Geometry check sheet. Reference: the model listing, model coordinates, mm. A direction names the side the tool comes from. Round coordinates to 2 decimals unless told otherwise and drop trailing zeros. Order: outer loops, then holes, each group sorted by start corner. A loop starts at its lowest first (then second) coordinate and runs counter-clockwise, first axis right, second up.
(1) Set-up check for faces 1 (the face through (13, -381, -39)), 2 (the face through (13, -193, 0)): record each of +Z, -Z, +X, -X, +Y, -Y from which the full face is reachable in a straight line by a thin tool's end or side.
(2) Release check for a two-part mould opening along Z. For faces 3 (the face through (12.522, -13.668, -42.964)), 4 (the face through (25.4, -168, -37)), 5 (the face through (13, -193, -76.2)) record: +Z half, -Z half, draft (parallel to the pull), parting line (faces both ways), or undercut.
(3) Sectioned sample at A-A (y = -25.4). Record the boundary of the cut face in (x, z), plus the area to 3 significant figures.
(4) Sectioned sample at D-D (z = -88). Record the boundary of the cut face in (x, y), plus the area to 3 significant figures.
(5) Sectioned sample at C-C (x = 14.5). Record the boundary of the cut face in (y, z), plus the area to 3 significant figures.
(6) Go/stop test with flat-tipped pins: pin 1 (12 mm diameter, centred on x = 6.5, y = -10.5, fed in from +Z); pin 2 (10 mm diameter, centred on x = 14, y = -322.5, fed in from -Z). Record where each tip stops, or that it passes through.
(7) Material ranges on line 1 along Z through (x, y) = (19.75, -25.4); line 2 along Z through (x, y) = (3, -243.5); line 3 along Z through (x, y) = (9.75, -14), recorded low to high.
(8) Sectioned sample at B-B (z = -38.1). Record the boundary of the cut face in (x, y), plus the area to 3 significant figures.
from build123d import *

# Parameters (mm, degrees)
F0_W     = 381
F0_H     = 76.2
F0_R     = 12.7
F1_DEPTH = 25.4


with BuildPart() as f1:
    # F0 (on Right) → F1 (new body)
    with BuildSketch(Plane.YZ):
        with Locations((-190.5, -38.1)):
            Rectangle(F0_W, F0_H)
        with Locations((-25.4, -38.1)):
            Circle(F0_R, mode=Mode.SUBTRACT)
        Polygon((50.8, 50.8), (0, 0), (0, -76.2), (50.8, -127), align=None)
    extrude(amount=F1_DEPTH)


solid = f1.part
Answer below:
1. face 1: +Z, -Z, +X, -X, -Y
1. face 2: +Z, +X, -X, -Y
2. face 3: undercut
2. face 4: draft
2. face 5: -Z half
3. outline: (0, -76.2) - (25.4, -76.2) - (25.4, -50.8) - (0, -50.8) - close; (0, -25.4) - (25.4, -25.4) - (25.4, 0) - (0, 0) - close
3. area: 1,290 mm2
4. outline: (0, 11.8) - (25.4, 11.8) - (25.4, 50.8) - (0, 50.8) - close
4. area: 991 mm2
5. outline: (-381, -76.2) - (0, -76.2) - (50.8, -127) - (50.8, 50.8) - (0, 0) - (-381, 0) - close; hole circle Ø25.4 at (-25.4, -38.1)
5. area: 35,000 mm2
6. pin 1: stops at z = 0
6. pin 2: stops at z = -76.2
7. line 1: z = -76.2 to -50.8, -25.4 to 0
7. line 2: z = -76.2 to 0
7. line 3: z = -76.2 to -43.7, -32.5 to 0
8. outline: (0, -381) - (25.4, -381) - (25.4, -38.1) - (0, -38.1) - close; (0, -12.7) - (25.4, -12.7) - (25.4, 50.8) - (0, 50.8) - close
8. area: 10,300 mm2
